```python
from build123d import *

# Parameters (mm, degrees)
F0_W = 1.6
F0_H = 28
F2_R = 1.8


with BuildPart() as f1:
    # F0 (on Front) → F1 (revolve)
    with BuildSketch(Plane.XZ):
        Polygon((-31.599971, 22.402998), (-26.6, 22.419994), (-25, 22.419994), (-25, 24.819994), (-28.2, 24.819994), align=None)
        with Locations((-25.8, 8.419994)):
            Rectangle(F0_W, F0_H)
    revolve(axis=Axis((0, 0, -8.381579), (0, 0, -1)))

    # F2
    f2_edges = [f1.edges().sort_by_distance(p)[0] for p in [
        (25, 0, 24.819994),
        (28.2, 0, 24.819994),
    ]]
    fillet(f2_edges, radius=F2_R)


solid = f1.part
```
The model under review builds one solid part; all positions refer to its coordinate system, in mm. A direction names the side the tool comes from. Round coordinates to 2 decimals unless told otherwise and drop trailing zeros. Loops run counter-clockwise (first coordinate to the right, second up) from the corner with the lowest first, then second, coordinate; pieces in that order, holes last. Notation, with made-up numbers: M 47.25,12.25 L 91.25,12.25 A23 ccw 91.25,24.25 Z; hole C -34,-34 d10. An arc over 180 degrees is marked long. Answer as a JSON object with one key per item and string values.
(1) Tool access review of faces 1 (the conical face through (-25.6, 8.06, 22.42)), 2 (the conical face through (6.254, -28.166, 24.357)): name each direction out of +Z, -Z, +X, -X, +Y, -Y from which nothing blocks a thin tool from reaching the whole face with its end or side.
Resolved:
{"face 1": "-Z", "face 2": "+Z"}
(2) To check wall thickness, follow line 1 along Y through (x, z) = (0, 3.5); line 2 along X through (y, z) = (-16, 4); line 3 along X through (y, z) = (9, 21). State the ranges of each line that lie inside material, in increasing order.
Resolved:
{"line 1": "-26.6 to -25, 25 to 26.6", "line 2": "-21.25 to -19.21, 19.21 to 21.25", "line 3": "-25.03 to -23.32, 23.32 to 25.03"}
(3) Draft analysis for pull direction Y (two halves, no side actions). For faces 3 (the cylindrical face through (-12.27, -23.6, 8.62)), 4 (the cylindrical face through (-23.846, 7.509, 8.92)), 5 (the flat face through (24, -8, -5.58)), state which applies: released by +Y, released by -Y, zero draft, split by the parting line, or undercut.
Resolved:
{"face 3": "split by the parting line", "face 4": "undercut", "face 5": "zero draft"}
(4) Clearance check with flat-ended pins moving along their axes: P1, Ø12, axis at x = -1.5, z = 1, coming from the -Y side; P2, Ø8, axis at y = 14.5, z = -2, coming from the +X side; P3, Ø1, axis at x = -19.5, z = 10, coming from the -Y side. State where each tip first meets the part, or that it passes through.
Resolved:
{"P1": "y = -26.6", "P2": "x = 24.44", "P3": "y = -18.62"}
(5) Take a section at A-A on y = 0. Give the boundary of the cut face in (x, z).
Resolved:
{"outline": "M -31.6,22.4 L -26.6,22.42 L -26.6,-5.58 L -25,-5.58 L -25,23.02 A1.8 ccw -26.8,24.82 L -27.63,24.82 A1.8 ccw -28.67,24.49 Z; M 25,-5.58 L 26.6,-5.58 L 26.6,22.42 L 31.6,22.4 L 28.67,24.49 A1.8 ccw 27.63,24.82 L 26.8,24.82 A1.8 ccw 25,23.02 Z"}
(6) Take a section at C-C on z = 0. Give the boundary of the cut face in (x, y).
Resolved:
{"outline": "C 0,0 d53.2; hole C 0,0 d50"}
